from build123d import *

# Parameters (mm, degrees)
SKETCH1_R                  = 41.275
SKETCH1_R_2                = 24.13
BOSS_EXTRUDE1_DEPTH        = 4.1275
F_3_4_3_4_DIAMETER_HOLE1_D = 3.4
CUT_EXTRUDE2_DEPTH         = 59.952491678
CIRPATTERN1_COUNT          = 3
F_3_4_3_4_DIAMETER_HOLE2_D = 3.4
SKETCH8_R                  = 3.175
CUT_EXTRUDE3_DEPTH         = 5.999999906


with BuildPart() as part:
    # Sketch1 → Boss-Extrude1 (new, symmetric)
    with BuildSketch(Plane.XY):
        Circle(SKETCH1_R)
        Circle(SKETCH1_R_2, mode=Mode.SUBTRACT)
    extrude(amount=BOSS_EXTRUDE1_DEPTH, both=True)

    # Ø3.4 (3.4) Diameter Hole1 (through all)
    with Locations(Plane.XY.offset(4.1275)):
        with Locations((-34.925, 0), (0, 34.925), (34.925, 0)):
            Hole(F_3_4_3_4_DIAMETER_HOLE1_D / 2)

    # Sketch5 → Cut-Extrude2 (cut, through all)
    with BuildSketch(Plane(origin=(0, 0, -4.1275), x_dir=(-1, 0, 0), z_dir=(0, 0, -1))):
        with BuildLine():
            Line((-23.096897519, 13.335), (0, 13.335))
            Line((0, 13.335), (0, -13.335))
            Line((0, -13.335), (-23.096897519, -13.335))
            ThreePointArc((-23.096897519, -13.335), (-26.67, 0), (-23.096897519, 13.335))
        make_face()
    cut_extrude2 = extrude(amount=-CUT_EXTRUDE2_DEPTH, mode=Mode.SUBTRACT)

    # CirPattern1: Cut-Extrude2 ×3 about axis
    cirpattern1_axis = Axis((0, 0, 0), (0, 0, 1))
    for i in range(1, CIRPATTERN1_COUNT):
        add(cut_extrude2.rotate(cirpattern1_axis, i * 360 / CIRPATTERN1_COUNT), mode=Mode.SUBTRACT)

    # Ø3.4 (3.4) Diameter Hole2 (through all)
    with Locations(Plane.XY.offset(4.1275)):
        with Locations((15.833393176, -33.954821241)):
            Hole(F_3_4_3_4_DIAMETER_HOLE2_D / 2)

    # Sketch8 → Cut-Extrude3 (cut)
    with BuildSketch(Plane.XY.offset(4.1275)):
        with Locations((0, 34.925)):
            Circle(SKETCH8_R)
        with Locations((34.925, 0)):
            Circle(SKETCH8_R)
        with Locations((15.833393176, -33.954821241)):
            Circle(SKETCH8_R)
        with Locations((-34.925, 0)):
            Circle(SKETCH8_R)
    extrude(amount=-CUT_EXTRUDE3_DEPTH, mode=Mode.SUBTRACT)


solid = part.part
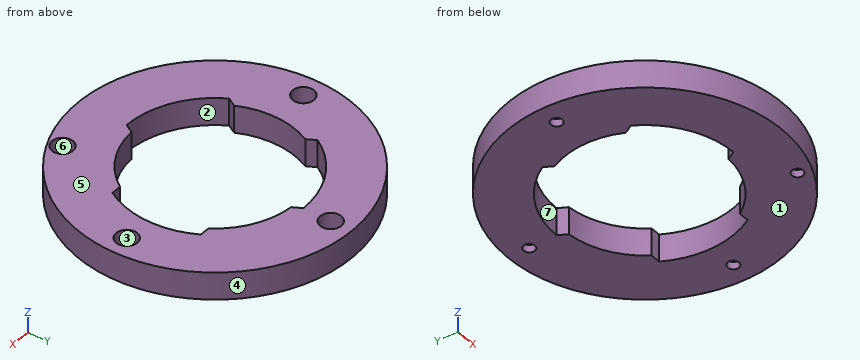
Read the model definition and answer for the solid it produces. Units are mm, in the model's axes. Face numbers are marked on the shaded views. A direction names the side the tool comes from. Round coordinates to 2 decimals unless told otherwise and drop trailing zeros. Write each loop counter-clockwise with the first axis right and the second up, starting at its lowest first coordinate (ties: lowest second). Pieces come first, ordered by that corner, then holes. Notation, with made-up numbers: M 74,5.5 L 124,5.5 A8 cw 124,20.5 Z; hole C 7.25,82.25 d8. An arc over 180 degrees is marked long. Use a Markdown table: item, result.
1) Straight lines are drawn through the part: line 1 along Y through (x, z) = (0, 1.7) (3 decimals); line 2 along Y through (x, z) = (14.5, -3.25); line 3 along Y through (x, z) = (-22, -3.5). For each, find the intervals that lie inside material, in ascending order. Write a range as [from, to].
Answers follow:
| item | result |
|---|---|
| line 1 | y = [-41.275, -26.67], [26.67, 31.75], [38.1, 41.275] |
| line 2 | y = [-38.64, -35.01], [-32.9, -19.29], [19.29, 38.64] |
| line 3 | y = [-34.92, -15.08], [-11.44, -9.91], [9.91, 11.44], [15.08, 34.92] |
2) The part is cut by section D-D (z = -0.5). Write down the section's boundary in (x, y) (3 decimals), plus the area to 3 significant figures.
Answers follow:
| item | result |
|---|---|
| outline | C 0,0 d82.55; hole C -34.925,0 d6.35; hole M -23.097,-13.335 A26.67 ccw 0,-26.67 L 1.493,-24.084 A24.13 ccw 20.111,-13.335 L 23.097,-13.335 A26.67 ccw 23.097,13.335 L 20.111,13.335 A24.13 ccw 1.493,24.084 L 0,26.67 A26.67 ccw -23.097,13.335 L -21.604,10.749 A24.13 ccw -21.604,-10.749 Z; hole C 0,34.925 d6.35; hole C 15.833,-33.955 d6.35; hole C 34.925,0 d6.35 |
| area | 3,180 mm2 |
3) The part is cut by section C-C (y = -19). Write down the section's boundary in (x, z), plus the area to 3 significant figures.
Answers follow:
| item | result |
|---|---|
| outline | M -36.64,-4.13 L -18.72,-4.13 L -18.72,4.13 L -36.64,4.13 Z; M 14.87,-4.13 L 36.64,-4.13 L 36.64,4.13 L 14.87,4.13 Z |
| area | 328 mm2 |
4) The part is cut by section B-B (x = 8). Write down the section's boundary in (y, z).
Answers follow:
| item | result |
|---|---|
| outline | M -40.49,-4.13 L -22.77,-4.13 L -22.77,4.13 L -40.49,4.13 Z; M 22.77,-4.13 L 40.49,-4.13 L 40.49,4.13 L 22.77,4.13 Z |
5) Flat-ended cylindrical pins translate along their axes: pin 1 (3 mm diameter, centred on x = 16, y = -35.5, fed in from +Z); pin 2 (3 mm diameter, centred on y = 12.5, z = 3, fed in from +X); pin 3 (2 mm diameter, centred on x = 0, y = 34.925, fed in from -Z); pin 4 (3.5 mm diameter, centred on x = 21, z = 0, fed in from -Y). Find the tip coordinate at first contact, or state that the pin passes through.
Answers follow:
| item | result |
|---|---|
| pin 1 | stops at z = -1.87 |
| pin 2 | stops at x = 39.78 |
| pin 3 | passes through |
| pin 4 | stops at y = -36.51 |
6) The part is cut by section A-A (y = 0). Give the number of separate pieces and of enclosed holes in the cut face, plus the area to 3 significant figures.
Answers follow:
| item | result |
|---|---|
| separate pieces | 4 |
| enclosed holes | 0 |
| area | 171 mm2 |
7) A tool of negligible diameter and unlimited length cuts with its end or side. For the marked faces 5, 6 and 7, from which of +Z, -Z, +X, -X, +Y, -Y can it reach the whole face along a straight path? Write none if from no direction.
Answers follow:
| item | result |
|---|---|
| face 5 | +Z, +X, -X, +Y, -Y |
| face 6 | +Z |
| face 7 | +Z, -Z |
8) For a pull along Y with two mould halves and no side action, classify the marked faces 1, 2, 3 and 4 as pulls with the +Y half, pulls with the -Y half, needs draft (parallel to the pull), parting line crosses it, or undercut.
Answers follow:
| item | result |
|---|---|
| face 1 | needs draft |
| face 2 | undercut |
| face 3 | undercut |
| face 4 | parting line crosses it |
